Model file for the job. Use its own axes, mm. Face numbers are marked on the shaded views. A direction names the side the tool comes from. Round coordinates to 2 decimals unless told otherwise and drop trailing zeros. Order: outer loops, then holes, each group sorted by start corner. A loop starts at its lowest first (then second) coordinate and runs counter-clockwise, first axis right, second up. Notation, with made-up numbers: (69, 55) - (112, 55) arc R9 ccw to (112, 63) - close; hole circle Ø6 at (-37, -25). An arc over 180 degrees is marked (long way). Write item = value, one per line. Start each with the question number.
from build123d import *

# Parameters (mm, degrees)
SKETCH_W     = 3.5
SKETCH_H     = 6.5
PAD002_DEPTH = 1.8
PAD003_DEPTH = 2.7
SKETCH004_W  = 1.5
SKETCH004_H  = 1.2
POCKET_DEPTH = 2.5
SKETCH005_W  = 7.5
SKETCH005_H  = 2.5
PAD004_DEPTH = 1.5
CHAMFER_SIZE = 1
SKETCH006_R  = 0.5
PAD005_DEPTH = 30
PAD001_DEPTH = 1.8
SKETCH002_W  = 20
SKETCH002_H  = 13
SKETCH002_R  = 1.5
PAD_DEPTH    = 1.8


with BuildPart() as pad005:
    # Sketch → Pad002 (new body)
    with BuildSketch(Plane(origin=(36, 1.65, 0), x_dir=(1, 0, 0), z_dir=(0, -1, 0))):
        with Locations((0, 3.25)):
            Rectangle(SKETCH_W, SKETCH_H)
    extrude(amount=PAD002_DEPTH)

    # Sketch003 → Pad003 (new body)
    with BuildSketch(Plane(origin=(36, 1.65, 0), x_dir=(1, 0, 0), z_dir=(0, 1, 0))):
        Polygon((-1.75, -0.6), (1.75, -0.6), (2.75, -1.6), (2.75, -6.5), (1.75, -7.5), (-1.75, -7.5), (-2.75, -6.5), (-2.75, -1.6), align=None)
    extrude(amount=PAD003_DEPTH)

    # Sketch004 → Pocket (cut)
    with BuildSketch(Plane(origin=(36, -0.15, 0), x_dir=(1, 0, 0), z_dir=(0, -1, 0))):
        with Locations((0, 3.5)):
            Rectangle(SKETCH004_W, SKETCH004_H)
    extrude(amount=-POCKET_DEPTH, mode=Mode.SUBTRACT)

    # Sketch005 → Pad004 (new body)
    with BuildSketch(Plane(origin=(36, -0.15, 0), x_dir=(1, 0, 0), z_dir=(0, -1, 0))):
        with Locations((0, 6.25)):
            Rectangle(SKETCH005_W, SKETCH005_H)
    extrude(amount=PAD004_DEPTH)

    # Chamfer
    chamfer_edges = [pad005.edges().sort_by_distance(p)[0] for p in [
        (33.25, 4.35, 4.05),
        (33.75, 4.35, 1.1),
        (36, 4.35, 0.6),
        (38.25, 4.35, 1.1),
        (38.75, 4.35, 4.05),
        (38.25, 4.35, 7),
        (36, 4.35, 7.5),
        (33.75, 4.35, 7),
    ]]
    chamfer(chamfer_edges, length=CHAMFER_SIZE)

    # Sketch006 → Pad005 (new body)
    with BuildSketch(Plane(origin=(39.75, 1.65, 0), x_dir=(0, 0, 1), z_dir=(1, 0, 0))):
        with Locations((6.25, 2.55)):
            Circle(SKETCH006_R)
    extrude(amount=-PAD005_DEPTH)


with BuildPart() as padcover:
    # Sketch001 → Pad001 (new body)
    with BuildSketch(Plane.XZ):
        Polygon((10, 0), (1.75, 0), (1.75, 6.5), (-1.75, 6.5), (-1.75, 0), (-10, 0), (-10, 12.5), (10, 12.5), align=None)
    extrude(amount=PAD001_DEPTH)


with BuildPart() as fusion:
    # Sketch002 → Pad (new body)
    with BuildSketch(Plane(origin=(21, 0, 0), x_dir=(1, 0, 0), z_dir=(0, -1, 0))):
        with Locations((0, 6.5)):
            Rectangle(SKETCH002_W, SKETCH002_H)
        with Locations((-4.3, 3.8)):
            Circle(SKETCH002_R, mode=Mode.SUBTRACT)
        with Locations((4.3, 3.8)):
            Circle(SKETCH002_R, mode=Mode.SUBTRACT)
    extrude(amount=PAD_DEPTH)

    # Fusion: union Pad005, PadCover
    add(pad005.part)
    add(padcover.part)


solid = fusion.part
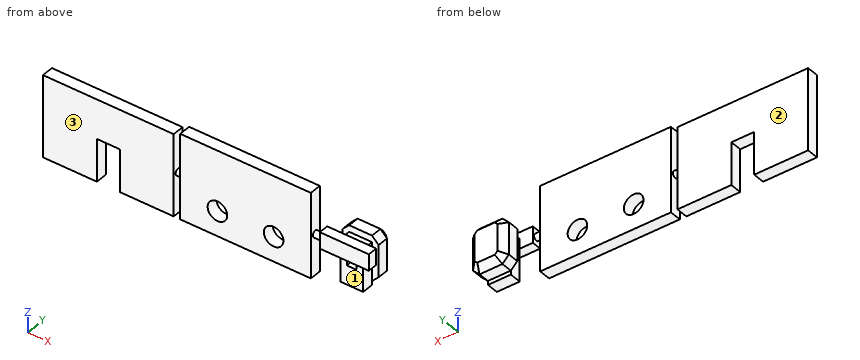
Item 1: Drop flat-ended pins along their axis: pin 1 (1 mm diameter, centred on x = 36, z = 3.5, fed in from -Y); pin 2 (2 mm diameter, centred on x = -0.5, y = -1, fed in from -Z); pin 3 (1.2 mm diameter, centred on x = 36, z = 7, fed in from -Y). Give the stop position or say it passes through.
Item 2: Probe L1, parallel to Z at x = 25.3, y = -1.3; L2, parallel to X at y = -0.25, z = 11.25; L3, parallel to X at y = -0.5, z = 3.5. List the from-to ranges inside material, lowest first.
Item 3: Saw through at A-A, the plane x = 16.7. Give the cut face in (y, z), then the cut area to 3 significant figures.
Item 4: Saw through at B-B, the plane z = 9. Give the cut face in (x, y).
Item 5: Saw through at D-D, the plane y = -0.9. Give the cut face in (x, z), then the cut area to 3 significant figures.
Item 6: Saw through at C-C, the plane y = 1. Give the cut face in (x, z).
Item 7: Which spindle directions (+Z, -Z, +X, -X, +Y, -Y) get a long thin tool onto all of the face, cutting with end or side? Do the marked faces 1, 2 and 3. Say none if no direction does.
Check sheet entries:
q1.pin_1 = 2.35
q1.pin_2 = 6.5
q1.pin_3 = -1.65
q2.L1 = 0 to 2.3, 5.3 to 13
q2.L2 = -10 to 10, 11 to 31
q2.L3 = -10 to -1.75, 1.75 to 10, 11 to 15.23, 18.17 to 23.83, 26.77 to 31
q3.outline = (-1.8, 0) - (0, 0) - (0, 2.3) - (-1.8, 2.3) - close; (-1.8, 5.3) - (0, 5.3) - (0, 13) - (-1.8, 13) - close
q3.area = 18.0 mm2
q4.outline = (-10, -1.8) - (10, -1.8) - (10, 0) - (-10, 0) - close; (11, -1.8) - (31, -1.8) - (31, 0) - (11, 0) - close
q5.outline = (-10, 0) - (-1.75, 0) - (-1.75, 6.5) - (1.75, 6.5) - (1.75, 0) - (10, 0) - (10, 5.75) - (11, 5.75) - (11, 0) - (31, 0) - (31, 5.75) - (32.25, 5.75) - (32.25, 5) - (39.75, 5) - (39.75, 7.5) - (32.25, 7.5) - (32.25, 6.75) - (31, 6.75) - (31, 13) - (11, 13) - (11, 6.75) - (10, 6.75) - (10, 12.5) - (-10, 12.5) - close; hole circle Ø3 at (16.7, 3.8); hole circle Ø3 at (25.3, 3.8)
q5.area = 494 mm2
q6.outline = (34.25, 0) - (37.75, 0) - (37.75, 6.5) - (34.25, 6.5) - close; hole (35.25, 2.9) - (36.75, 2.9) - (36.75, 4.1) - (35.25, 4.1) - close
q7.face_1 = -Z, +X, -Y
q7.face_2 = +Z, -Z, -X, +Y
q7.face_3 = +Z, -Z, +X, -X, -Y
